Design review of the part built by this model. Coordinates are the model's own, in mm. A direction names the side the tool comes from. Give positions to 0.01 mm unless a question says otherwise; leave off trailing zeros. Loops run counter-clockwise (first coordinate to the right, second up) from the corner with the lowest first, then second, coordinate; pieces in that order, holes last. Notation, with made-up numbers: (83, 65) -> (114, 65) arc R30 ccw to (114, 101) -> close; hole circle Ø7 at (-35, 59.25). An arc over 180 degrees is marked (long way). Answer as CSV lines item,"result".
Autodesk Inventor part; units mm, degrees
ref_plane "YZ Plane" through (0, 0, 0) normal (1, 0, 0) x (0, 1, 0)
ref_plane "XZ Plane" through (0, 0, 0) normal (0, 1, 0) x (-1, 0, 0)
ref_plane "XY Plane" through (0, 0, 0) normal (0, 0, 1) x (1, 0, 0)
sketch "Skizze1" plane through (0, 0, 0) normal (0, 0, 1) x (1, 0, 0)
  line L0 (52.3, 47.7) -> (-52.3, 47.7)
  arc A0 (-52.3, 47.7) -> (-54.3, 45.7) centre (-52.3, 45.7) ccw
  line L1 (54.3, 22.8) -> (54.3, 45.7)
  line L2 (-54.3, 45.7) -> (-54.3, -45.7)
  line L3 (-52.3, -47.7) -> (52.3, -47.7)
  arc A1 (-54.3, -45.7) -> (-52.3, -47.7) centre (-52.3, -45.7) ccw
  circle A2 centre (-50.8, -44.2) radius 1.5
  circle A3 centre (50.8, 44.2) radius 1.5
  arc A4 (52.3, -47.7) -> (54.3, -45.7) centre (52.3, -45.7) ccw
  line L4 (54.3, -45.7) -> (54.3, -8.2)
  line L5 (54.3, 22.8) -> (54.3, -8.2)
  arc A5 (54.3, 45.7) -> (52.3, 47.7) centre (52.3, 45.7) ccw
  circle A6 centre (-50.8, 44.2) radius 1.5
  circle A7 centre (50.8, -44.2) radius 1.5
  point P0 (0, 0)
extrude "Extrusion1" add sketch "Skizze1" along normal blind 7
sketch "Skizze2" plane through (0, 0, 0) normal (0, 0, -1) x (-1, 0, 0)
  line L0 (53.1, -44.5) -> (53.1, 44.5)
  line L1 (51.1, 46.5) -> (-51.1, 46.5)
  line L2 (-53.1, 44.5) -> (-53.1, -44.5)
  line L3 (-51.1, -46.5) -> (51.1, -46.5)
  line L4 (-51.3, -46.7) -> (51.3, -46.7)
  line L5 (53.3, -44.7) -> (53.3, 44.7)
  line L6 (51.3, 46.7) -> (-51.3, 46.7)
  line L7 (-53.3, 44.7) -> (-53.3, -44.7)
  line L8 (-53.3, -46.7) -> (53.3, 46.7) construction
  line L9 (53.3, -46.7) -> (-53.3, 46.7) construction
  arc A0 (53.3, 44.7) -> (51.3, 46.7) centre (51.3, 44.7) ccw
  arc A1 (-51.3, 46.7) -> (-53.3, 44.7) centre (-51.3, 44.7) ccw
  arc A2 (-53.3, -44.7) -> (-51.3, -46.7) centre (-51.3, -44.7) ccw
  arc A3 (51.3, -46.7) -> (53.3, -44.7) centre (51.3, -44.7) ccw
  line L10 (-56.7586, -49.6784) -> (56.7586, -49.6784)
  line L11 (56.7586, -49.6784) -> (56.7586, 49.6784)
  line L12 (56.7586, 49.6784) -> (-56.7586, 49.6784)
  line L13 (-56.7586, 49.6784) -> (-56.7586, -49.6784)
  line L14 (-56.7586, -49.6784) -> (56.7586, 49.6784) construction
  line L15 (56.7586, -49.6784) -> (-56.7586, 49.6784) construction
  point P0 (0, 0)
  dimension "d2" = 0.2
  dimension "d3" = 0.2
  dimension "d4" = 2
extrude "Extrusion2" cut sketch "Skizze2" against normal blind 1.85
sketch "Skizze3" plane through (0, 0, 0) normal (0, 0, -1) x (-1, 0, 0)
  line L0 (-50.7142, 40.2858) -> (-46.8858, 44.1142)
  arc A0 (-45.4716, 44.7) -> (-46.8858, 44.1142) centre (-45.4716, 42.7) ccw
  line L1 (-45.4716, 44.7) -> (45.4716, 44.7)
  arc A1 (-50.7142, 40.2858) -> (-51.3, 38.8716) centre (-49.3, 38.8716) ccw
  line L2 (-51.3, -38.8716) -> (-51.3, 38.8716)
  line L3 (50.7142, -40.2858) -> (46.8858, -44.1142)
  arc A2 (50.7142, -40.2858) -> (51.3, -38.8716) centre (49.3, -38.8716) ccw
  line L4 (51.3, 38.8716) -> (51.3, -38.8716)
  arc A3 (45.4716, -44.7) -> (46.8858, -44.1142) centre (45.4716, -42.7) ccw
  line L5 (45.4716, -44.7) -> (-45.4716, -44.7)
  arc A4 (51.3, 38.8716) -> (50.7142, 40.2858) centre (49.3, 38.8716) ccw
  line L6 (46.8858, 44.1142) -> (50.7142, 40.2858)
  arc A5 (46.8858, 44.1142) -> (45.4716, 44.7) centre (45.4716, 42.7) ccw
  arc A6 (-46.8858, -44.1142) -> (-45.4716, -44.7) centre (-45.4716, -42.7) ccw
  line L7 (-46.8858, -44.1142) -> (-50.7142, -40.2858)
  arc A7 (-51.3, -38.8716) -> (-50.7142, -40.2858) centre (-49.3, -38.8716) ccw
  circle A8 centre (-50.8, -44.2) radius 1.5
  circle A9 centre (-50.8, 44.2) radius 1.5
  circle A10 centre (50.8, 44.2) radius 1.5
  circle A11 centre (50.8, -44.2) radius 1.5
  point P0 (0, 0)
extrude "Extrusion3" cut sketch "Skizze3" against normal blind 5 contours L0 A0 L1 A5 L6 A4 L4 A2 L3 A3 L5 A6 L7 A7 L2 A1
sketch "Skizze4" plane through (54.3, -45.7, 7) normal (1, 0, 0) x (0, 0, -1)
  line L0 (3.15, 38) -> (3.15, 68.5)
  line L1 (0, 0) -> (0, 91.4)
  line L2 (7, 90.4) -> (7, 1)
  line L3 (5.15, -2) -> (0, -2)
  line L4 (3.15, 68.5) -> (7, 68.5)
  line L5 (7, 1) -> (7, 90.4)
  line L6 (3.15, 38) -> (7, 38)
  line L7 (7, 68.5) -> (7, 38)
  point P0 (7, 45.7)
  dimension "d11" = 3.85
  dimension "d13" = 30.5
  dimension "d14" = 40
extrude "Extrusion4" cut sketch "Skizze4" against normal up to next
sketch "Skizze5" plane through (0, 0, 7) normal (0, 0, 1) x (1, 0, 0)
  circle A0 centre (-50.8, 44.2) radius 1.5
  circle A1 centre (-50.8, 44.2) radius 2.7
  line L0 (52.3, 47.7) -> (-52.3, 47.7)
  circle A2 centre (50.8, 44.2) radius 1.5
  circle A3 centre (50.8, 44.2) radius 2.5
  line L1 (-51.3, 46.7) -> (51.3, 46.7)
  circle A4 centre (50.8, -44.2) radius 1.5
  circle A5 centre (50.8, -44.2) radius 2.7
  line L2 (54.3, -45.7) -> (54.3, 45.7)
  circle A6 centre (-50.8, -44.2) radius 1.5
  circle A7 centre (-50.8, -44.2) radius 2.5
  line L3 (51.3, -46.7) -> (-51.3, -46.7)
  point P0 (0, 0)
  dimension "d17" = 0.8
  dimension "d18" = 0.8
extrude "Extrusion5" cut sketch "Skizze5" against normal blind 4
sketch "Skizze6" plane through (0, 0, 7) normal (0, 0, 1) x (1, 0, 0)
  line L0 (-27.7, 38.2) -> (25.3, 38.2)
  line L1 (25.3, 38.2) -> (25.3, 27.2)
  line L2 (25.3, 27.2) -> (-27.7, 27.2)
  line L3 (-27.7, 27.2) -> (-27.7, 38.2)
  line L4 (54.3, -45.7) -> (54.3, 45.7)
  line L5 (52.3, 47.7) -> (-52.3, 47.7)
  point P0 (0, 0)
  dimension "d21" = 53
  dimension "d22" = 11
  dimension "d23" = 29
  dimension "d24" = 9.5
extrude "Extrusion6" cut sketch "Skizze6" against normal up to next
properties part number "case rear" material "ABS-Kunststoff"
Q1. The part is to be moulded in two halves that separate along X. For faces 4 (the flat face through (53, 7, 3.85)), 5 (the cylindrical face through (-52.943, 42.557, 5.028)), 6 (the flat face through (-49.6, 43, 3)), 7 (the flat face through (54.3, -0.6, 4.4)), say which applies: pulls with the +X half, pulls with the -X half, needs draft (parallel to the pull), parting line crosses it, or undercut.
Filled sheet:
face 4,"needs draft"
face 5,"undercut"
face 6,"undercut"
face 7,"pulls with the +X half"
Q2. Clearance check with flat-ended pins moving along their axes: pin 1 Ø2.5 at (x, y) = (-50, -44.5) entering from +Z; pin 2 Ø0.9 at (y, z) = (33.5, 0.5) entering from +X; pin 3 Ø0.9 at (x, z) = (-24.5, 0.5) entering from -Y. State where each tip first meets the part, or that it passes through.
Filled sheet:
pin 1,"stops at z = 3"
pin 2,"stops at x = 53.3"
pin 3,"stops at y = -46.7"
Q3. We need section B-B, the plane x = 41. State the section outline as (y, z) points.
Filled sheet:
outline,"(-47.7, 1.85) -> (-46.7, 1.85) -> (-46.7, 0) -> (-44.7, 0) -> (-44.7, 5) -> (44.7, 5) -> (44.7, 0) -> (46.7, 0) -> (46.7, 1.85) -> (47.7, 1.85) -> (47.7, 7) -> (-47.7, 7) -> close"
Q4. For faces 1 (the cylindrical face through (53.375, -43.389, 5.028)), 2 (the flat face through (52, -7.7, 2)), 3 (the flat face through (-51.3, 1, 2)), list the 3-axis set-ups (+Z, -Z, +X, -X, +Y, -Y) from which the entire face can be reached by the end or side of a thin tool; tool diameter is ignored.
Filled sheet:
face 1,"+Z"
face 2,"-Z, +X"
face 3,"-Z"
Q5. To check wall thickness, follow probe 1 along Y at (x, z) = (-50.8, 5.6); probe 2 along X at (y, z) = (44.2, 5.9); probe 3 along X at (y, z) = (-13.5, 2.75). State the ranges of each line that lie inside material, in increasing order. Write a range as from..to.
Filled sheet:
probe 1,"y = -47.7..-46.7, -41.7..41.5, 46.9..47.7"
probe 2,"x = -54.3..-53.5, -48.1..48.3, 53.3..54.3"
probe 3,"x = -54.3..-51.3, 51.3..54.3"
Q6. We need section A-A, the plane y = -22.5. State the section outline as (x, z) points.
Filled sheet:
outline,"(-54.3, 1.85) -> (-53.3, 1.85) -> (-53.3, 0) -> (-51.3, 0) -> (-51.3, 5) -> (51.3, 5) -> (51.3, 0) -> (53.3, 0) -> (53.3, 1.85) -> (54.3, 1.85) -> (54.3, 7) -> (-54.3, 7) -> close"
Q7. We need section C-C, the plane y = 13. State the section outline as (x, z) points.
Filled sheet:
outline,"(-54.3, 1.85) -> (-53.3, 1.85) -> (-53.3, 0) -> (-51.3, 0) -> (-51.3, 5) -> (51.3, 5) -> (51.3, 3.85) -> (54.3, 3.85) -> (54.3, 7) -> (-54.3, 7) -> close"
